Geometry: see drawing. Coordinates: mm, zero at the bounding-box minimum. Round coordinates to 2 decimals unless told otherwise and drop trailing zeros. Loops run counter-clockwise (first coordinate to the right, second up) from the corner with the lowest first, then second, coordinate; pieces in that order, holes last.
(1) Material intervals for probe 1 along X at (y, z) = (65.7, 12.25); probe 2 along Z at (x, y) = (3.75, 66.1); probe 3 along Z at (x, y) = (12.25, 42), sorted ascending.
(2) Section D-D, the plane x = 22. Return the cut outline in (y, z), plus the area to 3 significant figures.
(3) Section A-A, the plane x = 12.25. Return the cut outline in (y, z), plus the area to 3 significant figures.
(4) First-contact query: pin 1 Ø5 at (y, z) = (28.5, 19) entering from -X; pin 2 Ø1.2 at (x, y) = (12, 66.5) entering from +Z; pin 3 Ø12 at (y, z) = (36.5, 4.5) entering from -X. Flat tips, straight axial feed; report the tip coordinate or a pass-through.
(5) Section C-C, the plane y = 20. Return the cut outline in (x, z).
(6) Mould query, pull axis Z, two halves, no side actions, for the marked faces 1, 2 and 3. Classes: pulls with the +Z half, pulls with the -Z half, needs draft (parallel to the pull), parting line crosses it, or undercut.
(7) Section B-B, the plane z = 13.75. Return the cut outline in (x, y), plus the area to 3 significant figures.
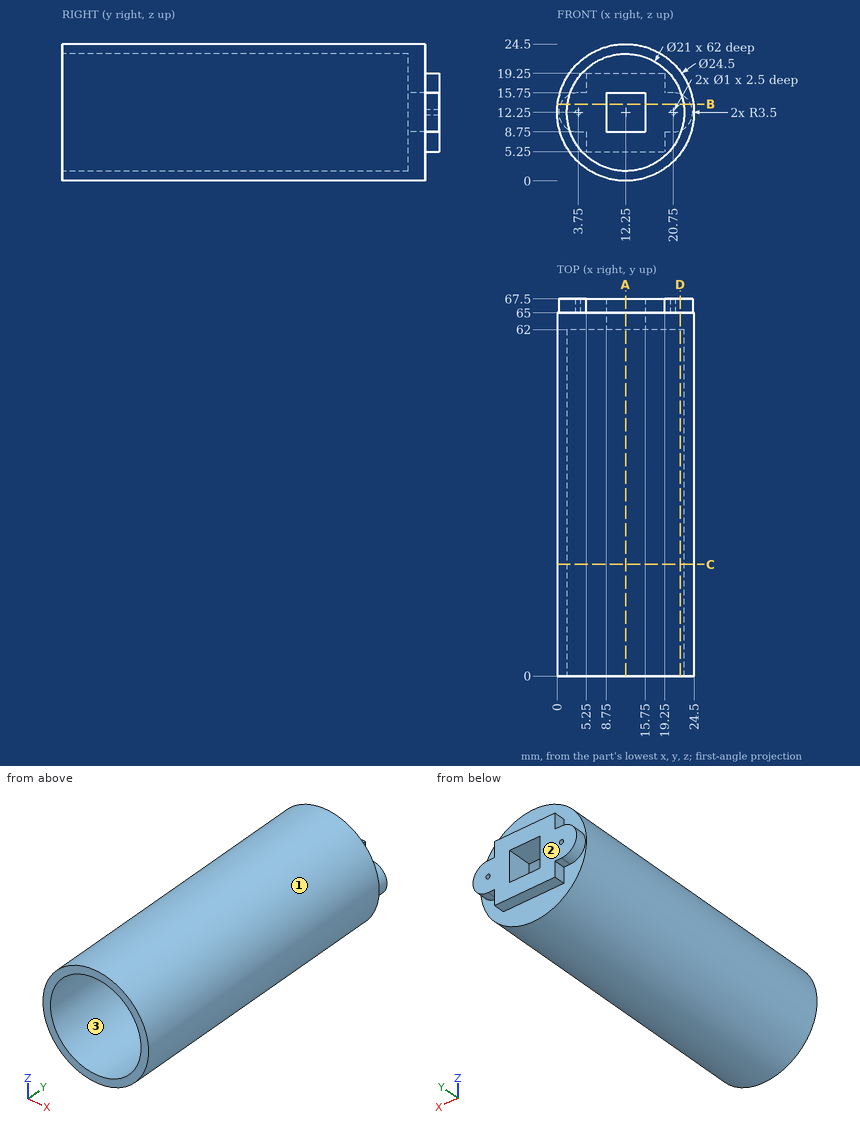
Output values:
1. probe 1: x = 0.25 to 3.25, 4.25 to 8.75, 15.75 to 20.25, 21.25 to 24.25
1. probe 2: z = 8.75 to 11.75, 12.75 to 15.75
1. probe 3: z = 0 to 1.75, 22.75 to 24.5
2. outline: (0, 4.83) - (65, 4.83) - (65, 8.98) - (67.5, 8.98) - (67.5, 15.52) - (65, 15.52) - (65, 19.67) - (0, 19.67) - (0, 16.15) - (62, 16.15) - (62, 8.35) - (0, 8.35) - close
2. area: 497 mm2
3. outline: (0, 0) - (65, 0) - (65, 5.25) - (67.5, 5.25) - (67.5, 8.75) - (62, 8.75) - (62, 1.75) - (0, 1.75) - close; (0, 22.75) - (62, 22.75) - (62, 15.75) - (67.5, 15.75) - (67.5, 19.25) - (65, 19.25) - (65, 24.5) - (0, 24.5) - close
3. area: 287 mm2
4. pin 1: stops at x = 0.76
4. pin 2: stops at z = 19.25
4. pin 3: stops at x = 0.13
5. outline: circle Ø24.5 at (12.25, 12.25); hole circle Ø21 at (12.25, 12.25)
6. face 1: parting line crosses it
6. face 2: needs draft
6. face 3: undercut
7. outline: (0.09, 0) - (1.86, 0) - (1.86, 62) - (8.75, 62) - (8.75, 67.5) - (0.59, 67.5) - (0.59, 65) - (0.09, 65) - close; (15.75, 62) - (22.64, 62) - (22.64, 0) - (24.41, 0) - (24.41, 65) - (23.91, 65) - (23.91, 67.5) - (15.75, 67.5) - close
7. area: 312 mm2
